from build123d import *

# Parameters (mm, degrees)
EXTRUDE_1_DEPTH          = 4
SKETCH_3_R               = 2
SKETCH_3_W               = 41
SKETCH_3_H               = 20
CUT_EXTRUDE_3_DEPTH      = 25
PATTERN_CIRCULAR_1_COUNT = 6


with BuildPart() as part:
    # 草图1 → 凸台-拉伸1 (new body)
    with BuildSketch(Plane(origin=(0, 0, 0), x_dir=(1, 0, 0), z_dir=(0, 1, 0))):
        with BuildLine():
            Line((78.581168228, 15), (78.581168228, -15))
            ThreePointArc((78.581168228, -15), (59.197125657, -34.177476433), (52.280965171, -60.553287944))
            Line((52.280965171, -60.553287944), (26.300203057, -75.553287944))
            ThreePointArc((26.300203057, -75.553287944), (0, -68.354952867), (-26.300203057, -75.553287944))
            Line((-26.300203057, -75.553287944), (-52.280965171, -60.553287944))
            ThreePointArc((-52.280965171, -60.553287944), (-59.197125657, -34.177476433), (-78.581168228, -15))
            Line((-78.581168228, -15), (-78.581168228, 15))
            ThreePointArc((-78.581168228, 15), (-59.197125657, 34.177476433), (-52.280965171, 60.553287944))
            Line((-52.280965171, 60.553287944), (-26.300203057, 75.553287944))
            ThreePointArc((-26.300203057, 75.553287944), (0, 69.054660136), (26.300203057, 75.553287944))
            Line((26.300203057, 75.553287944), (52.280965171, 60.553287944))
            ThreePointArc((52.280965171, 60.553287944), (59.197125657, 34.177476433), (78.581168228, 15))
        make_face()
    extrude(amount=EXTRUDE_1_DEPTH)

    # 草图3 → 切除-拉伸3 (cut, symmetric)
    with BuildSketch(Plane(origin=(0, 0, 0), x_dir=(1, 0, 0), z_dir=(0, 1, 0))):
        with Locations(Location((68.581168228, 5, 0), (0, 0, 270))):
            Circle(SKETCH_3_R)
        with Locations(Location((68.581168228, -5, 0), (0, 0, 270))):
            Circle(SKETCH_3_R)
        with Locations(Location((19.581168228, 5, 0), (0, 0, 270))):
            Circle(SKETCH_3_R)
        with Locations(Location((19.581168228, -5, 0), (0, 0, 270))):
            Circle(SKETCH_3_R)
        with Locations((44.081168228, 0)):
            Rectangle(SKETCH_3_W, SKETCH_3_H)
    cut_extrude_3 = extrude(amount=CUT_EXTRUDE_3_DEPTH, both=True, mode=Mode.SUBTRACT)

    # 阵列(圆周)1: 切除-拉伸3 ×6 about axis
    pattern_circular_1_axis = Axis((0, 0, 0), (0, 1, 0))
    for i in range(1, PATTERN_CIRCULAR_1_COUNT):
        add(cut_extrude_3.rotate(pattern_circular_1_axis, i * 360 / PATTERN_CIRCULAR_1_COUNT), mode=Mode.SUBTRACT)


solid = part.part
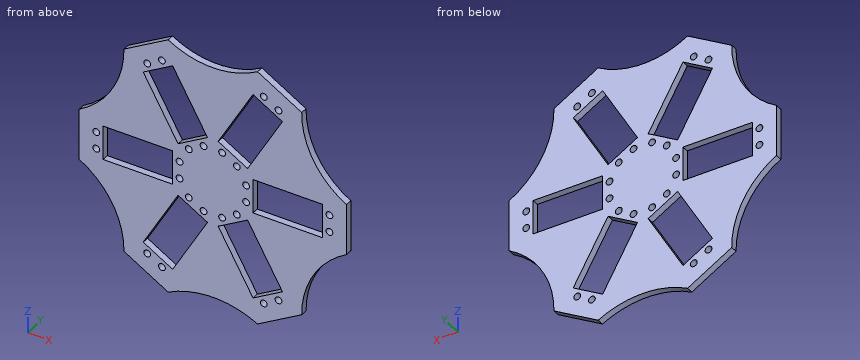
Design review of the part built by this model. Coordinates are the model's own, in mm. Give positions to 0.01 mm unless a question says otherwise; leave off trailing zeros. Order: outer loops, then holes, each group sorted by start corner. A loop starts at its lowest first (then second) coordinate and runs counter-clockwise, first axis right, second up. Notation, with made-up numbers: (33.5, -35) - (79.5, -35) arc R15 ccw to (79.5, -29) - close; hole circle Ø11 at (-26, 81.5). An arc over 180 degrees is marked (long way). Write item = value, one per line. Start each with the question number.
Q1. To check wall thickness, follow L1, parallel to X at y = 2.35, z = -24.5; L2, parallel to X at y = 2.5, z = -45.5; L3, parallel to Z at x = 37.5, y = 0.3. State the ranges of each line that lie inside material, in increasing order. Write a range as from..to.
Q2. We need section C-C on z = -30.5. State the section outline as (x, y) points, plus the area to 3 significant figures.
Q3. We need section D-D on y = 1.3. State how many separate pieces and enclosed holes the cut face has, plus the area to 3 significant figures.
Q4. Clearance check with flat-ended pins moving along their axes: pin 1 Ø2 at (x, y) = (-11.5, 2.5) entering from -Z; pin 2 Ø2 at (x, y) = (-61, 3) entering from +Z; pin 3 Ø2.5 at (x, z) = (14.12, 14.46) entering from +Y; pin 4 Ø2 at (x, y) = (-35.5, 1) entering from -Z. State where each tip first meets the part, or that it passes through.
Q5. We need section A-A on z = -5. State the section outline as (x, y) points, plus the area to 3 significant figures.
Q6. We need section B-B on x = 57. State the section outline as (y, z) points.
Working result:
q1.L1 = -66.41..-25.69, -4.73..4.73, 25.69..66.41
q1.L2 = -54.36..-37.82, -14.72..14.72, 37.82..54.36
q1.L3 = -69.09..-58.55, -55.24..-52.92, -44.95..-10, 10..44.95, 52.92..55.24, 58.55..69.09
q2.outline = (-61.53, 0) - (-29.16, 0) - (-29.16, 4) - (-61.53, 4) - close; (-6.06, 0) - (6.06, 0) - (6.06, 4) - (-6.06, 4) - close; (29.16, 0) - (61.53, 0) - (61.53, 4) - (29.16, 4) - close
q2.area = 308 mm²
q3.separate_pieces = 1
q3.enclosed_holes = 30
q3.area = 12,300 mm²
q4.pin_1 = -70.46
q4.pin_2 = 32.83
q4.pin_3 = through
q4.pin_4 = -70.82
q5.outline = (-78.58, 0) - (-70.58, 0) - (-70.58, 4) - (-78.58, 4) - close; (-66.58, 0) - (-64.58, 0) - (-64.58, 4) - (-66.58, 4) - close; (-23.58, 0) - (-21.58, 0) - (-21.58, 4) - (-23.58, 4) - close; (-17.58, 0) - (17.58, 0) - (17.58, 4) - (-17.58, 4) - close; (21.58, 0) - (23.58, 0) - (23.58, 4) - (21.58, 4) - close; (64.58, 0) - (66.58, 0) - (66.58, 4) - (64.58, 4) - close; (70.58, 0) - (78.58, 0) - (78.58, 4) - (70.58, 4) - close
q5.area = 237 mm²
q6.outline = (0, -38.43) - (4, -38.43) - (4, -10) - (0, -10) - close; (0, 10) - (4, 10) - (4, 38.43) - (0, 38.43) - close
